Source: CAD feature listing. Evaluate the final solid. Frame: model axes, mm. A direction names the side the tool comes from. Coordinates: 2 decimals unless noted, no trailing zeros. Order: outer loops, then holes, each group sorted by start corner. A loop starts at its lowest first (then second) coordinate and runs counter-clockwise, first axis right, second up. Notation, with made-up numbers: (66, -31) - (110, -31) arc R20 ccw to (110, 8) - close; hole circle Ø8 at (7.5, 40). An arc over 180 degrees is marked (long way). One line per question, with ' | ' between items. Start each with the question number.
(1) Section B-B (x = 16). Return the cut outline in (y, z).
(2) Section D-D (y = 22.5). Return the cut outline in (x, z), then the cut area to 3 significant figures.
(3) Line query: line 1 along X through (y, z) = (14.35, -4.25); line 2 along X through (y, z) = (4.5, -5.75). Output: solid intervals per line, ascending.
(4) Section C-C (z = -7.5). Return the cut outline in (x, y).
(5) Section A-A (z = -4.25). Return the cut outline in (x, y), then the cut area to 3 significant figures.
(6) Draft query along Z for faces 1 (the flat face through (10, 19, -4)), 2 (the flat face through (10, 10, -8.5)), 3 (the cylindrical face through (-1.61, 14.51, -5.25)). Return one class per face: +Z half, -Z half, draft (parallel to the pull), parting line (faces both ways), or undercut.
(7) Access query for faces 4 (the flat face through (20.2, 18, -4)), 5 (the flat face through (10, 10, 0)), 6 (the flat face through (0, 7, -4)), 7 (the flat face through (-3, 15, -4)). Directions: +Z, -Z, +X, -X, +Y, -Y. A direction counts if a zero-diameter tool reaches every point of the face in a straight line with its end or side. Return the directions, or none.
(8) Contact query for flat-ended pins moving along their axis: P1, Ø4.5, axis at x = 23, z = -3, coming from the +Y side; P2, Ø2, axis at y = 15.5, z = -6.5, coming from the +X side; P3, Ø1.2, axis at x = 21.85, z = -4.25, coming from the +Y side; P4, Ø2.5, axis at y = 6, z = -3.5, coming from the +X side. Output: stop coordinate, or through.
from build123d import *

# Parameters (mm, degrees)
SKETCH1_W           = 20.2
SKETCH1_H           = 8.5
BOSS_EXTRUDE1_DEPTH = 14
BOSS_EXTRUDE2_DEPTH = 1
SKETCH3_W           = 20.2
SKETCH3_H           = 8.5
BOSS_EXTRUDE3_DEPTH = 5.2
CUT_EXTRUDE1_DEPTH  = 20.2
SKETCH5_R           = 1
CUT_EXTRUDE2_DEPTH  = 32.280345267
SKETCH6_R           = 1.5
BOSS_EXTRUDE4_DEPTH = 4.8


with BuildPart() as part:
    # Sketch1 → Boss-Extrude1 (new body)
    with BuildSketch(Plane(origin=(0, 0, 0), x_dir=(1, 0, 0), z_dir=(0, 1, 0))):
        with Locations((10.1, 4.25)):
            Rectangle(SKETCH1_W, SKETCH1_H)
    extrude(amount=BOSS_EXTRUDE1_DEPTH)

    # Sketch2 → Boss-Extrude2 (add)
    with BuildSketch(Plane(origin=(0, 14, 0), x_dir=(1, 0, 0), z_dir=(0, 1, 0))):
        with BuildLine():
            Line((-1.65, 8.5), (21.85, 8.5))
            ThreePointArc((21.85, 8.5), (26.1, 4.25), (21.85, 0))
            Line((21.85, 0), (-1.65, 0))
            ThreePointArc((-1.65, 0), (-5.9, 4.25), (-1.65, 8.5))
        make_face()
    extrude(amount=BOSS_EXTRUDE2_DEPTH)

    # Sketch3 → Boss-Extrude3 (add)
    with BuildSketch(Plane(origin=(0, 15, 0), x_dir=(1, 0, 0), z_dir=(0, 1, 0))):
        with Locations((10.1, 4.25)):
            Rectangle(SKETCH3_W, SKETCH3_H)
    extrude(amount=BOSS_EXTRUDE3_DEPTH)

    # Sketch4 → Cut-Extrude1 (cut)
    with BuildSketch(Plane.XY):
        Polygon((0, 17), (7, 18.5), (10, 18.5), (10, 20.2), (20.2, 20.2), (20.2, 17.6), (23.419390589, 17.6), (23.419390589, 23.763762674), (-0.815558956, 23.763762674), align=None)
    extrude(amount=-CUT_EXTRUDE1_DEPTH, mode=Mode.SUBTRACT)

    # Sketch5 → Cut-Extrude2 (cut, through all)
    with BuildSketch(Plane(origin=(0, 15, 0), x_dir=(1, 0, 0), z_dir=(0, 1, 0))):
        with Locations(Location((-1.65, 4.25, 0), (0, 0, 270))):
            Circle(SKETCH5_R)
        with Locations(Location((21.85, 4.25, 0), (0, 0, 270))):
            Circle(SKETCH5_R)
    extrude(amount=-CUT_EXTRUDE2_DEPTH, mode=Mode.SUBTRACT)

    # Sketch6 → Boss-Extrude4 (add)
    with BuildSketch(Plane(origin=(0, 20.2, 0), x_dir=(1, 0, 0), z_dir=(0, 1, 0))):
        with Locations(Location((16, 4.25, 0), (0, 0, 90))):
            Circle(SKETCH6_R)
    extrude(amount=BOSS_EXTRUDE4_DEPTH)


solid = part.part
Response values:
1) outline: (0, -8.5) - (20.2, -8.5) - (20.2, -5.75) - (25, -5.75) - (25, -2.75) - (20.2, -2.75) - (20.2, 0) - (0, 0) - close
2) outline: circle Ø3 at (16, -4.25) | area: 7.07 mm²
3) line 1: x = -5.9 to -2.65, -0.65 to 20.85, 22.85 to 26.1 | line 2: x = 0 to 20.2
4) outline: (-4.39, 14) - (0, 14) - (0, 0) - (20.2, 0) - (20.2, 14) - (24.59, 14) - (24.59, 15) - (20.2, 15) - (20.2, 20.2) - (10, 20.2) - (10, 18.5) - (7, 18.5) - (0, 17) - (0, 15) - (-4.39, 15) - close
5) outline: (-5.9, 14) - (-2.65, 14) - (-2.65, 15) - (-5.9, 15) - close; (-0.65, 14) - (0, 14) - (0, 0) - (20.2, 0) - (20.2, 14) - (20.85, 14) - (20.85, 15) - (20.2, 15) - (20.2, 20.2) - (17.5, 20.2) - (17.5, 25) - (14.5, 25) - (14.5, 20.2) - (10, 20.2) - (10, 18.5) - (7, 18.5) - (0, 17) - (0, 15) - (-0.65, 15) - close; (22.85, 14) - (26.1, 14) - (26.1, 15) - (22.85, 15) - close | area: 408 mm²
6) face 1: draft | face 2: -Z half | face 3: undercut
7) face 4: +Z, -Z, +X, +Y | face 5: +Z, +X, -X, +Y, -Y | face 6: +Z, -Z, -X, -Y | face 7: +Z, -Z, -X, +Y
8) P1: stops at y = 15 | P2: stops at x = 25.87 | P3: passes through | P4: stops at x = 20.2
